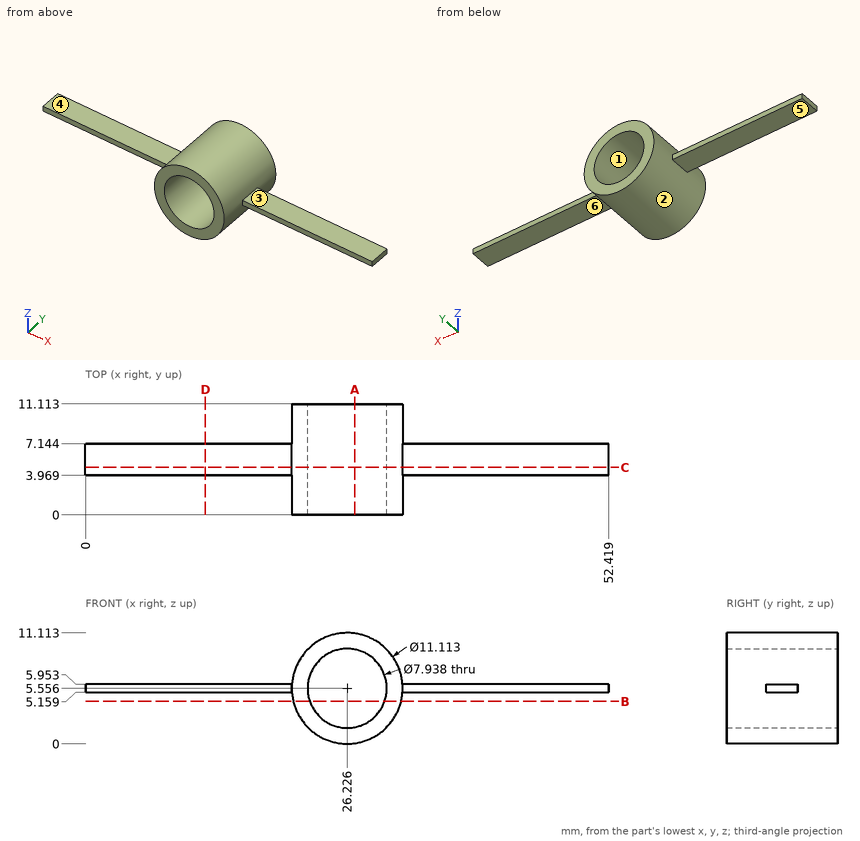
Drawing for the job (mm, zero at the part's lowest x, y, z). A direction names the side the tool comes from. Give positions to 0.01 mm unless a question says otherwise; leave off trailing zeros. Order: outer loops, then holes, each group sorted by start corner. A loop starts at its lowest first (then second) coordinate and runs counter-clockwise, first axis right, second up. Notation, with made-up numbers: M 17.25,38 L 36.25,38 A6 ccw 36.25,43 Z; hole C -7,-10.5 d9. An arc over 180 degrees is marked long. Put each result on its own line as item: value. Start each with the question number.
(1) Saw through at C-C, the plane y = 4.75. Write the cut outline in (x, z) (1 decimal).
(2) Which spindle directions (+Z, -Z, +X, -X, +Y, -Y) get a long thin tool onto all of the face, cutting with end or side? Do the marked faces 4, 5 and 6. Say none if no direction does.
(3) Mould opens along X. For the marked faces 1, 2 and 3 say: +X half, -X half, draft (parallel to the pull), parting line (faces both ways), or undercut.
(4) Flat gauge pins, fed straight in: pin 1 Ø1 at (y, z) = (7.5, 8) entering from -X; pin 2 Ø2.5 at (x, y) = (6.5, 6) entering from -Z; pin 3 Ø6 at (x, y) = (40.5, 4.5) entering from +Z. Where does each tip first touch, or does it go through?
(5) Saw through at B-B, the plane z = 4.25. Write the cut outline in (x, y) (1 decimal).
(6) Saw through at A-A, the plane x = 27. Write the cut outline in (y, z) (1 decimal).
(7) Drill centre lines: line 1 along X through (y, z) = (3.25, 5.5); line 2 along X through (y, z) = (4.75, 5.75); line 3 along Z through (x, y) = (49, 4.5). Where is each one in solid material? Low to high.
(8) Saw through at D-D, the plane x = 12. Write the cut outline in (y, z).
Check result:
1. outline: M 0,5.2 L 20.7,5.2 A5.6 ccw 31.8,5.2 L 52.4,5.2 L 52.4,6 L 31.8,6 A5.6 ccw 20.7,6 L 0,6 Z; hole C 26.2,5.6 d7.9
2. face 4: +Z, -X, +Y, -Y
2. face 5: -Z, -X, +Y, -Y
2. face 6: -Z, +X, +Y, -Y
3. face 1: undercut
3. face 2: parting line
3. face 3: draft
4. pin 1: stops at x = 21.02
4. pin 2: stops at z = 5.16
4. pin 3: stops at z = 5.95
5. outline: M 20.8,0 L 22.5,0 L 22.5,11.1 L 20.8,11.1 Z; M 30,0 L 31.6,0 L 31.6,11.1 L 30,11.1 Z
6. outline: M 0,0.1 L 11.1,0.1 L 11.1,1.7 L 0,1.7 Z; M 0,9.4 L 11.1,9.4 L 11.1,11.1 L 0,11.1 Z
7. line 1: x = 20.67 to 22.26, 30.19 to 31.78
7. line 2: x = 0 to 22.26, 30.19 to 52.42
7. line 3: z = 5.16 to 5.95
8. outline: M 3.97,5.16 L 7.14,5.16 L 7.14,5.95 L 3.97,5.95 Z
